Model file for the job. Use its own axes, mm. A direction names the side the tool comes from. Round coordinates to 2 decimals unless told otherwise and drop trailing zeros. Loops run counter-clockwise (first coordinate to the right, second up) from the corner with the lowest first, then second, coordinate; pieces in that order, holes last. Notation, with made-up numbers: M 65,-12 L 112,-12 A27 cw 112,7 Z; hole C 79,20 d1. An arc over 180 degrees is marked long. Use a Markdown table: item, result. Add a question column.
Item 1: Wall check: L1, parallel to Z at x = 4.25, y = 0; L2, parallel to Y at x = 11, z = 0; L3, parallel to X at y = 3.5, z = -12. Give the ranges that are in metal, low to high. Write a range as from..to.
Item 2: Saw through at A-A on x = 1.75. Write the cut outline in (y, z), then the cut area to 3 significant figures.
Item 3: Pin check, flat tips, straight feed: P1, Ø5, axis at x = 7, y = -10.5, coming from the -Z side; P2, Ø3, axis at x = 10, z = -5.5, coming from the +Y side; P3, Ø6, axis at x = 11.5, z = -11.5, coming from the -Y side; P4, Ø11, axis at y = 0, z = 0, coming from the +X side. Stop position of each tip, or through.
Item 4: Saw through at B-B on x = 7.25. Write the cut outline in (y, z).
Item 5: Tool access for faces 1 (the flat face through (15.9, -14, 0)), 2 (the flat face through (15.6, -9.2, 3.2)), 3 (the flat face through (0.3, -9.2, -3.2)): list every direction of +Z, -Z, +X, -X, +Y, -Y with a clear straight run to the whole face (end or side of a thin tool).
Item 6: Two-plate mould, pull along Z, no slides. Class faces 4 (the cylindrical face through (8, 0, -6)), 5 (the cylindrical face through (2.259, 10.648, -13.887)), 6 (the flat face through (15.9, -7, -2)): +Z half, -Z half, draft (parallel to the pull), parting line (faces both ways), or undercut.
```python
from build123d import *

# Parameters (mm, degrees)
F2_SIZE = 0.5
F3_SIZE = 1


with BuildPart() as f1:
    # F0 (on Front) → F1 (revolve)
    with BuildSketch(Plane.XZ):
        with BuildLine():
            Line((0, 9.2), (0, 6))
            Line((0, 6), (15.9, 6))
            Line((15.9, 6), (15.9, 9.2))
            Line((15.9, 9.2), (15.6, 9.5))
            Line((15.6, 9.5), (15.6, 13.5))
            Line((15.6, 13.5), (15.9, 13.8))
            Line((15.9, 13.8), (15.9, 17.5))
            Line((15.9, 17.5), (11.832976, 17.5))
            ThreePointArc((11.832976, 17.5), (7.95, 15.65), (4.067024, 17.5))
            Line((4.067024, 17.5), (0, 17.5))
            Line((0, 17.5), (0, 13.8))
            Line((0, 13.8), (0.3, 13.5))
            Line((0.3, 13.5), (0.3, 9.5))
            Line((0.3, 9.5), (0, 9.2))
        make_face()
    revolve(axis=Axis((29.48505, 0, 0), (1, 0, 0)))

    # F2
    f2_edges = [f1.edges().sort_by_distance(p)[0] for p in [
        (0, 0, -17.5),
        (15.9, 0, -17.5),
    ]]
    chamfer(f2_edges, length=F2_SIZE)

    # F3
    f3_edges = [f1.edges().sort_by_distance(p)[0] for p in [
        (15.9, 0, -6),
        (0, 0, -6),
    ]]
    chamfer(f3_edges, length=F3_SIZE)


solid = f1.part
```
Entries:
| question | item | result |
|---|---|---|
| 1 | L1 | -17.29..-6, 6..17.29 |
| 1 | L2 | -16.69..-6, 6..16.69 |
| 1 | L3 | 0.3..15.6 |
| 2 | outline | C 0,0 d35; hole C 0,0 d12 |
| 2 | area | 849 mm2 |
| 3 | P1 | z = -13.96 |
| 3 | P2 | y = 16.3 |
| 3 | P3 | y = -15.29 |
| 3 | P4 | through |
| 4 | outline | C 0,0 d31.4; hole C 0,0 d12 |
| 5 | face 1 | +Z, -Z, +X, +Y, -Y |
| 5 | face 2 | +X |
| 5 | face 3 | -X |
| 6 | face 4 | undercut |
| 6 | face 5 | parting line |
| 6 | face 6 | draft |
